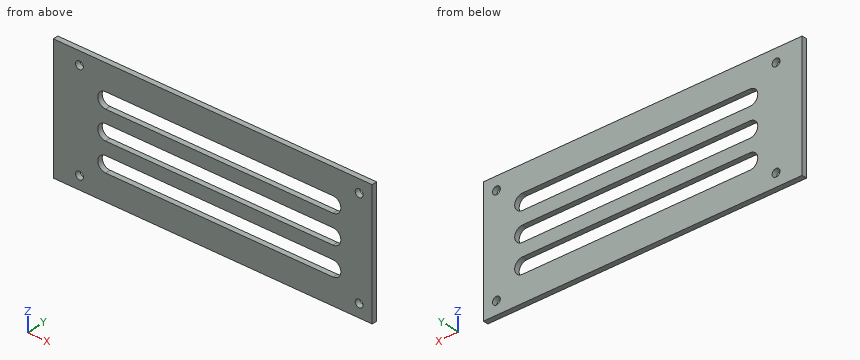
```python
from build123d import *

# Parameters (mm, degrees)
SKETCH_1_W          = 122
SKETCH_1_H          = 48
SKETCH_1_R          = 1.5
EXTRUDE_1_DEPTH     = 2
CUT_EXTRUDE_1_DEPTH = 120.987499349


with BuildPart() as part:
    # 草图1 → 凸台-拉伸1 (new body)
    with BuildSketch(Plane(origin=(0, 0, 0), x_dir=(1, 0, 0), z_dir=(0, 1, 0))):
        with Locations((51, 19)):
            Rectangle(SKETCH_1_W, SKETCH_1_H)
        with Locations(Location((0, 38, 0), (0, 0, 270))):
            Circle(SKETCH_1_R, mode=Mode.SUBTRACT)
        with Locations(Location((0, 0, 0), (0, 0, 270))):
            Circle(SKETCH_1_R, mode=Mode.SUBTRACT)
        with Locations(Location((107, 38, 0), (0, 0, 270))):
            Circle(SKETCH_1_R, mode=Mode.SUBTRACT)
        with Locations(Location((107, 0, 0), (0, 0, 270))):
            Circle(SKETCH_1_R, mode=Mode.SUBTRACT)
    extrude(amount=EXTRUDE_1_DEPTH)

    # 草图2 → 切除-拉伸1 (cut, through all)
    with BuildSketch(Plane(origin=(0, 2, 0), x_dir=(1, 0, 0), z_dir=(0, 1, 0))):
        with BuildLine():
            Line((10, 33), (97, 33))
            ThreePointArc((97, 33), (100, 30), (97, 27))
            Line((97, 27), (10, 27))
            ThreePointArc((10, 27), (7, 30), (10, 33))
        make_face()
        with BuildLine():
            Line((10, 16), (97, 16))
            ThreePointArc((97, 16), (100, 19), (97, 22))
            Line((97, 22), (10, 22))
            ThreePointArc((10, 22), (7, 19), (10, 16))
        make_face()
        with BuildLine():
            Line((10, 5), (97, 5))
            ThreePointArc((97, 5), (100, 8), (97, 11))
            Line((97, 11), (10, 11))
            ThreePointArc((10, 11), (7, 8), (10, 5))
        make_face()
    extrude(amount=-CUT_EXTRUDE_1_DEPTH, mode=Mode.SUBTRACT)


solid = part.part
```
CAD build for the part. Positions are in the model's coordinates, mm. Round coordinates to 2 decimals unless told otherwise and drop trailing zeros. Order: outer loops, then holes, each group sorted by start corner. A loop starts at its lowest first (then second) coordinate and runs counter-clockwise, first axis right, second up. Notation, with made-up numbers: (-8.75, 83.25) - (11.25, 83.25) arc R22 cw to (11.25, 117.25) - close; hole circle Ø3 at (45.5, 55). An arc over 180 degrees is marked (long way). Answer in a Markdown table with one row per item. Add a question column.
(1) Band-saw the part on D-D on z = -8. List the corners of the cut face in (x, y).
(2) Band-saw the part on B-B on y = 0.3. List the corners of the cut face in (x, z).
(3) Band-saw the part on C-C on x = 73. List the corners of the cut face in (y, z), and give its area (3 significant figures).
(4) Probe L1, parallel to Z at x = 107, y = 0.5; L2, parallel to Z at x = 42, y = 0.7; L3, parallel to X at y = 1.2, z = 0. List the from-to ranges inside material, lowest first. Write a range as [from, to].
(5) Band-saw the part on A-A on z = 0. List the corners of the cut face in (x, y).
Data:
| question | item | result |
|---|---|---|
| 1 | outline | (-10, 0) - (7, 0) - (7, 2) - (-10, 2) - close; (100, 0) - (112, 0) - (112, 2) - (100, 2) - close |
| 2 | outline | (-10, -43) - (112, -43) - (112, 5) - (-10, 5) - close; hole circle Ø3 at (0, -38); hole circle Ø3 at (0, 0); hole (10, -33) - (97, -33) arc R3 ccw to (97, -27) - (10, -27) arc R3 ccw to start; hole (10, -22) - (97, -22) arc R3 ccw to (97, -16) - (10, -16) arc R3 ccw to start; hole (10, -11) - (97, -11) arc R3 ccw to (97, -5) - (10, -5) arc R3 ccw to start; hole circle Ø3 at (107, -38); hole circle Ø3 at (107, 0) |
| 3 | outline | (0, -43) - (2, -43) - (2, -33) - (0, -33) - close; (0, -27) - (2, -27) - (2, -22) - (0, -22) - close; (0, -16) - (2, -16) - (2, -11) - (0, -11) - close; (0, -5) - (2, -5) - (2, 5) - (0, 5) - close |
| 3 | area | 60.0 mm^2 |
| 4 | L1 | z = [-43, -39.5], [-36.5, -1.5], [1.5, 5] |
| 4 | L2 | z = [-43, -33], [-27, -22], [-16, -11], [-5, 5] |
| 4 | L3 | x = [-10, -1.5], [1.5, 105.5], [108.5, 112] |
| 5 | outline | (-10, 0) - (-1.5, 0) - (-1.5, 2) - (-10, 2) - close; (1.5, 0) - (105.5, 0) - (105.5, 2) - (1.5, 2) - close; (108.5, 0) - (112, 0) - (112, 2) - (108.5, 2) - close |
